```python
from build123d import *

# Parameters (mm, degrees)
F0_R          = 12.7
F0_R_2        = 9.525
F1_DEPTH      = 12.7
F1_DEPTH_BACK = 12.7
F2_W          = 254
F2_H          = 71.842049
F3_DEPTH      = 12.7
F4_R          = 9.525
F5_DEPTH      = 38.1


with BuildPart() as f1:
    # F0 (on Right) → F1 (new body, two sides)
    with BuildSketch(Plane.YZ) as f1_sk:
        with BuildLine():
            Line((-71.842049, 0), (0, 0))
            Line((0, 0), (110.580256, 110.580256))
            ThreePointArc((110.580256, 110.580256), (114.700433, 113.33327), (119.560512, 114.3))
            Line((119.560512, 114.3), (413.839488, 114.3))
            ThreePointArc((413.839488, 114.3), (418.699567, 113.33327), (422.819744, 110.580256))
            Line((422.819744, 110.580256), (593.180256, -59.780256))
            ThreePointArc((593.180256, -59.780256), (597.300433, -62.53327), (602.160512, -63.5))
            Line((602.160512, -63.5), (638.081537, -63.5))
            ThreePointArc((638.081537, -63.5), (649.814807, -55.66008), (647.061793, -41.819744))
            Line((647.061793, -41.819744), (443.861793, 161.380256))
            ThreePointArc((443.861793, 161.380256), (439.741616, 164.13327), (434.881537, 165.1))
            Line((434.881537, 165.1), (396.781537, 165.1))
            Line((396.781537, 165.1), (339.497045, 264.31965))
            Line((339.497045, 264.31965), (193.902955, 264.31965))
            Line((193.902955, 264.31965), (136.618463, 165.1))
            Line((136.618463, 165.1), (98.518463, 165.1))
            ThreePointArc((98.518463, 165.1), (93.658384, 164.13327), (89.538207, 161.380256))
            Line((89.538207, 161.380256), (-71.842049, 0))
        make_face()
        with Locations((607.421024, -38.1)):
            Circle(F0_R, mode=Mode.SUBTRACT)
        with Locations((165.1, 139.7)):
            Circle(F0_R_2, mode=Mode.SUBTRACT)
        with Locations((190.5, 139.7)):
            Circle(F0_R_2, mode=Mode.SUBTRACT)
        with Locations((215.9, 139.7)):
            Circle(F0_R_2, mode=Mode.SUBTRACT)
        with Locations((241.3, 139.7)):
            Circle(F0_R_2, mode=Mode.SUBTRACT)
        with Locations((266.7, 139.7)):
            Circle(F0_R_2, mode=Mode.SUBTRACT)
        Polygon((352.787446, 165.1), (180.612554, 165.1), (215.9, 226.21965), (317.5, 226.21965), align=None, mode=Mode.SUBTRACT)
        with Locations((292.1, 139.7)):
            Circle(F0_R_2, mode=Mode.SUBTRACT)
        with Locations((317.5, 139.7)):
            Circle(F0_R_2, mode=Mode.SUBTRACT)
        with Locations((342.9, 139.7)):
            Circle(F0_R_2, mode=Mode.SUBTRACT)
        with Locations((368.3, 139.7)):
            Circle(F0_R_2, mode=Mode.SUBTRACT)
    extrude(amount=F1_DEPTH)
    extrude(f1_sk.sketch, amount=-F1_DEPTH_BACK)

    # F2 (on Top) → F3 (join)
    with BuildSketch(Plane.XY):
        with Locations((0, -35.921025)):
            Rectangle(F2_W, F2_H)
    extrude(amount=-F3_DEPTH)

    # F4 (on face) → F5 (join)
    with BuildSketch(Plane(origin=(0, 0, -12.7), x_dir=(1, 0, 0), z_dir=(0, 0, -1))):
        with Locations((76.2, 52.792049)):
            Circle(F4_R)
        with Locations((-76.2, 52.792049)):
            Circle(F4_R)
    extrude(amount=F5_DEPTH)


solid = f1.part
```
The listing builds one solid part. Answer for the finished solid, in the listing's coordinates (mm). A direction names the side the tool comes from. Give positions to 0.01 mm unless a question says otherwise; leave off trailing zeros. Write each loop counter-clockwise with the first axis right and the second up, starting at its lowest first coordinate (ties: lowest second). Pieces come first, ordered by that corner, then holes. Notation, with made-up numbers: (66, -15.75) - (100, -15.75) arc R26 cw to (100, 2.25) - close; hole circle Ø9 at (88, -14). An arc over 180 degrees is marked (long way). Use one line per item in the form item = value. Start each with the question number.
1) Find section C-C on z = 183. Determine the outline of the cut face in (x, y), plus the area to 3 significant figures.
2) Find section D-D on y = 368.3. Determine the outline of the cut face in (x, z) (3 decimals).
3) The mould has two halves that part along Y. Classify faces 5 (the face through (0.18, 9.98, 81.82)), 6 (the face through (0.2, 506.8, 26.6)), 7 (the face through (-127, -36, -6)): pulls with the +Y half, pulls with the -Y half, needs draft (parallel to the pull), parting line crosses it, or undercut.
4) Flat-ended cylindrical pins translate along their axes: pin 1 Ø3 at (x, y) = (2, 328) entering from -Z; pin 2 Ø2 at (y, z) = (428, 135.5) entering from +X; pin 3 Ø22 at (y, z) = (292.1, 139.7) entering from -X. Find the tip coordinate at first contact, or state that the pin passes through.
5) Consider line 1 along Z through (x, y) = (-4, 317); line 2 along Z through (x, y) = (-2, 342); line 3 along X through (y, z) = (575.5, 19). Determine where each line is inside the solid, lowest interval first. Write a range as from..to.
6) Find section A-A on y = 266.7. Determine the outline of the cut face in (x, z) (3 decimals), plus the area to 3 significant figures.
7) A tool of negligible diameter and unlimited length cuts with its end or side. For faces 1 (the face through (-30, -35, 0)), 2 (the face through (0, 265, 114.3)), 3 (the face through (80.595, -44.342, -31.483)), 4 (the face through (0, 416, 165.1)), from which of +Z, -Z, +X, -X, +Y, -Y can it reach the whole face along a straight path? Write none if from no direction.
8) Find section B-B on x = 76.2. Determine the outline of the cut face in (y, z).
Geometry results:
q1.outline = (-12.7, 146.95) - (12.7, 146.95) - (12.7, 190.95) - (-12.7, 190.95) - close; (-12.7, 342.45) - (12.7, 342.45) - (12.7, 386.45) - (-12.7, 386.45) - close
q1.area = 2,230 mm2
q2.outline = (-12.7, 114.3) - (12.7, 114.3) - (12.7, 130.175) - (-12.7, 130.175) - close; (-12.7, 149.225) - (12.7, 149.225) - (12.7, 214.431) - (-12.7, 214.431) - close
q3.face_5 = pulls with the -Y half
q3.face_6 = undercut
q3.face_7 = needs draft
q4.pin_1 = 114.3
q4.pin_2 = 12.7
q4.pin_3 = -12.7
q5.line_1 = 114.3..130.19, 149.21..165.1, 226.22..264.32
q5.line_2 = 114.3..130.22, 149.18..165.1, 183.78..259.98
q5.line_3 = -12.7..12.7
q6.outline = (-12.7, 114.3) - (12.7, 114.3) - (12.7, 130.175) - (-12.7, 130.175) - close; (-12.7, 149.225) - (12.7, 149.225) - (12.7, 165.1) - (-12.7, 165.1) - close; (-12.7, 226.22) - (12.7, 226.22) - (12.7, 264.32) - (-12.7, 264.32) - close
q6.area = 1,770 mm2
q7.face_1 = +Z, -X, +Y, -Y
q7.face_2 = -Z, +X, -X
q7.face_3 = -Z
q7.face_4 = +Z, +X, -X, +Y
q8.outline = (-71.84, -12.7) - (-62.32, -12.7) - (-62.32, -50.8) - (-43.27, -50.8) - (-43.27, -12.7) - (0, -12.7) - (0, 0) - (-71.84, 0) - close
